Check sheet for the modelled part. Datum: model origin and axes. Units: mm. A direction names the side the tool comes from. Round coordinates to 2 decimals unless told otherwise and drop trailing zeros. Write each loop counter-clockwise with the first axis right and the second up, starting at its lowest first coordinate (ties: lowest second). Pieces come first, ordered by that corner, then holes.
Item 1: Section check A-A, the plane x = 0. Record the cut outline in (y, z).
Item 2: Section check B-B, the plane y = 7.75. Record the cut outline in (x, z).
Item 3: Set-up check for faces 1 (the flat face through (4, 10, 23)), 2 (the cylindrical face through (8.621, 3.498, -34.497)), 3 (the cylindrical face through (-0.521, 8.428, -28.495)), 4 (the flat face through (0, 6.9, 35)), 5 (the cylindrical face through (-17.879, 8.428, 22.195)): record each of +Z, -Z, +X, -X, +Y, -Y from which the full face is reachable in a straight line by a thin tool's end or side.
Item 4: Depth check by flat-ended pin: pin 1 (1.9 mm diameter, centred on x = -20, z = 28, fed in from +Y); pin 2 (3.5 mm diameter, centred on x = 8, z = 33, fed in from +Y); pin 3 (3 mm diameter, centred on x = 7, y = 6.5, fed in from -Z). Enter the tip coordinate at first touch or a pass-through.
Item 5: Section check D-D, the plane y = 3.5. Record the cut outline in (x, z), plus the area to 3 significant figures.
Item 6: Material ranges on line 1 along Z through (x, y) = (0, 5.25); line 2 along X through (y, z) = (4.25, -28); line 3 along Z through (x, y) = (-20, 2), recorded low to high.
Item 7: Section check C-C, the plane z = -33. Record the cut outline in (x, y).
Item 8: Release check for a two-part mould opening along X. For faces 6 (the cylindrical face through (7.513, 3.498, 31.454)), 7 (the flat face through (13, 0, 18)), 8 (the cylindrical face through (18.26, 8.43, 21.88)), 9 (the cylindrical face through (-19.014, 3.498, -26.714)) record: pulls with the +X half, pulls with the -X half, needs draft (parallel to the pull), parting line crosses it, or undercut.
Autodesk Inventor part; units mm, degrees
ref_plane "YZ Plane" through (0, 0, 0) normal (1, 0, 0) x (0, 1, 0)
ref_plane "XZ Plane" through (0, 0, 0) normal (0, 1, 0) x (-1, 0, 0)
ref_plane "XY Plane" through (0, 0, 0) normal (0, 0, 1) x (1, 0, 0)
sketch "Skizze1" plane through (0, 0, 0) normal (0, 1, 0) x (-1, 0, 0)
  line L0 (-27.5, 29.0474) -> (-27.5, -29.0474)
  line L1 (27.5, -29.0474) -> (27.5, 29.0474)
  arc A0 (27.5, 29.0474) -> (-27.5, 29.0474) centre (0, 0) ccw
  arc A1 (-27.5, -29.0474) -> (27.5, -29.0474) centre (0, 0) ccw
  dimension "d4" = 27.5
  dimension "d5" = 40
extrude "Basebody 1" add sketch "Skizze1" along normal blind 6.9
sketch "Skizze2" plane through (0, 6.9, 0) normal (0, 1, 0) x (1, 0, 0)
  line L0 (-27.5, 29.0474) -> (-27.5, -29.0474)
  arc A0 (27.5, 29.0474) -> (-27.5, 29.0474) centre (0, 0) ccw
  line L1 (-27.5, -7.4833) -> (-27.5, 7.4833)
  arc A1 (-27.5, -29.0474) -> (27.5, -29.0474) centre (0, 0) ccw
  line L2 (27.5, -7.4833) -> (27.5, 7.4833)
  arc A2 (-27.5, -7.4833) -> (27.5, -7.4833) centre (0, 0) ccw
  arc A3 (27.5, 7.4833) -> (-27.5, 7.4833) centre (0, 0) ccw
extrude "Basebody 2" add sketch "Skizze2" along normal blind 3.1
sketch "Skizze3" plane through (0, 10, 0) normal (0, 1, 0) x (1, 0, 0)
  arc A0 (27.5, 29.0474) -> (-27.5, 29.0474) centre (0, 0) ccw
  circle A1 centre (0, 0) radius 22
  dimension "d11" = 44
extrude "44H7 Drill" cut sketch "Skizze3" against normal through all
sketch "Skizze4" plane through (0, 0, 0) normal (0, 1, 0) x (-1, 0, 0)
  circle A0 centre (0, 30) radius 2.5
  arc A1 (27.5, 7.4833) -> (-27.5, 7.4833) centre (0, 0) ccw
  dimension "d14" = 30
  dimension "d15" = 5
extrude "5H7 Drill" cut sketch "Skizze4" along normal through all
sketch "Skizze6" plane through (0, 0, 0) normal (0, 1, 0) x (-1, 0, 0)
  circle A0 centre (20, 28) radius 2
  line L0 (-27.5, 29.0474) -> (-27.5, -29.0474)
  circle A1 centre (-8, 33) radius 2
  line L1 (32.1852, 0) -> (-31.2523, 0)
  circle A2 centre (20, -28) radius 2
  circle A3 centre (-8, -33) radius 2
  point P0 (0, 0)
  dimension "d18" = 4
  dimension "d19" = 28
  dimension "d20" = 47.5
  dimension "d21" = 4
  dimension "d22" = 33
  dimension "d23" = 19.5
hole "M4" at (8, 0, 33) at (-20, 0, 28) at (-20, 0, -28) at (8, 0, -33) direction (0, 1, 0) diameter 3.242 end through all
chamfer "Fasen2" distance 1 angle 45 1 edges at (-22, 10, 0)
properties part number "27-30-400 Bearing, Housing Measuring Head" material "Aluminium"
Values found:
1. outline: (0, -40) - (6.9, -40) - (6.9, -28.5) - (10, -28.5) - (10, -23) - (9, -22) - (0, -22) - close; (0, 22) - (9, 22) - (10, 23) - (10, 27.5) - (0, 27.5) - close; (0, 32.5) - (6.9, 32.5) - (6.9, 40) - (0, 40) - close
2. outline: (-27.5, -7.48) arc R28.5 ccw to (27.5, -7.48) - (27.5, 7.48) arc R28.5 ccw to (1.95, 28.43) arc R2.5 cw to (-1.95, 28.43) arc R28.5 ccw to (-27.5, 7.48) - close; hole circle Ø44 at (0, 0)
3. face 1: +Z, -Z, +X, -X, +Y
3. face 2: +Y, -Y
3. face 3: -Z, +Y
3. face 4: +Z, +Y
3. face 5: +Z, -X, +Y
4. pin 1: passes through
4. pin 2: stops at y = 6.9
4. pin 3: stops at z = -39.62
5. outline: (-27.5, -29.05) arc R40 ccw to (27.5, -29.05) - (27.5, 29.05) arc R40 ccw to (-27.5, 29.05) - close; hole circle Ø44 at (0, 0); hole circle Ø3.24 at (-20, -28); hole circle Ø3.24 at (-20, 28); hole circle Ø5 at (0, 30); hole circle Ø3.24 at (8, -33); hole circle Ø3.24 at (8, 33)
5. area: 2,450 mm2
6. line 1: z = -40 to -22, 22 to 27.5, 32.5 to 40
6. line 2: x = -27.5 to -21.62, -18.38 to 27.5
6. line 3: z = -34.64 to -29.62, -26.38 to -9.17, 9.17 to 26.38, 29.62 to 34.64
7. outline: (-22.61, 0) - (6.38, 0) - (6.38, 6.9) - (-22.61, 6.9) - close; (9.62, 0) - (22.61, 0) - (22.61, 6.9) - (9.62, 6.9) - close
8. face 6: undercut
8. face 7: needs draft
8. face 8: pulls with the +X half
8. face 9: undercut
